Geometry: final body of the model. Coordinates: model frame, mm. A direction names the side the tool comes from. Give positions to 0.01 mm unless a question says otherwise; leave off trailing zeros. Loops run counter-clockwise (first coordinate to the right, second up) from the corner with the lowest first, then second, coordinate; pieces in that order, holes last. Notation, with made-up numbers: (69.5, 26) - (85.5, 26) arc R8 cw to (85.5, 30) - close; hole circle Ø1 at (66.5, -6.5). An arc over 180 degrees is marked (long way). Answer in a Markdown table with one row per item.
from build123d import *

# Parameters (mm, degrees)
CYLINDER004_R     = 2.4
CYLINDER004_DEPTH = 35
CYLINDER011_R     = 2
CYLINDER011_DEPTH = 40
CYLINDER008_R     = 3.15
CYLINDER008_DEPTH = 16
BOX006_W          = 10
BOX006_H          = 24
BOX006_DEPTH      = 15
CHAMFER004_SIZE   = 3
CHAMFER017_SIZE   = 0.4
BOX004_W          = 7
BOX004_H          = 7.8
BOX004_DEPTH      = 8
CHAMFER010_SIZE   = 0.4
BOX003_W          = 18
BOX003_H          = 42
BOX003_DEPTH      = 8
CHAMFER_SIZE      = 7
CHAMFER015_SIZE   = 10
FILLET004_R       = 1
BOX_W             = 1
BOX_H             = 7.8
BOX_DEPTH         = 15


with BuildPart() as cylinder004:
    # Cylinder004 → Cylinder004 (new body)
    with BuildSketch(Plane(origin=(9, 15, 0), x_dir=(1, 0, 0), z_dir=(0, 0, 1))):
        Circle(CYLINDER004_R)
    extrude(amount=CYLINDER004_DEPTH)


with BuildPart() as cylinder011:
    # Cylinder011 → Cylinder011 (new body)
    with BuildSketch(Plane(origin=(9, 34, 2), x_dir=(1, 0, 0), z_dir=(0, 0, 1))):
        Circle(CYLINDER011_R)
    extrude(amount=CYLINDER011_DEPTH)


with BuildPart() as cylinder008:
    # Cylinder008 → Cylinder008 (new body)
    with BuildSketch(Plane(origin=(-2, 15, -7.5), x_dir=(0, 0, -1), z_dir=(1, 0, 0))):
        Circle(CYLINDER008_R)
    extrude(amount=CYLINDER008_DEPTH)


with BuildPart() as chamfer017:
    # Box006 → Box006 (new body)
    with BuildSketch(Plane(origin=(0, 3, -15), x_dir=(1, 0, 0), z_dir=(0, 0, 1))):
        with Locations((5, 12)):
            Rectangle(BOX006_W, BOX006_H)
    extrude(amount=BOX006_DEPTH)

    # Chamfer004
    chamfer004_edges = [chamfer017.edges().sort_by_distance(p)[0] for p in [
        (5, 3, -15),
        (5, 27, -15),
    ]]
    chamfer(chamfer004_edges, length=CHAMFER004_SIZE)

    # Chamfer017
    chamfer017_edges = [chamfer017.edges().sort_by_distance(p)[0] for p in [
        (10, 3, -6),
        (10, 4.5, -13.5),
        (10, 15, -15),
        (10, 27, -6),
        (10, 25.5, -13.5),
    ]]
    chamfer(chamfer017_edges, length=CHAMFER017_SIZE)


with BuildPart() as chamfer010:
    # Box004 → Box004 (new body)
    with BuildSketch(Plane(origin=(-7, 11.1, 0), x_dir=(1, 0, 0), z_dir=(0, 0, 1))):
        with Locations((3.5, 3.9)):
            Rectangle(BOX004_W, BOX004_H)
    extrude(amount=BOX004_DEPTH)

    # Chamfer010
    chamfer010_edges = [chamfer010.edges().sort_by_distance(p)[0] for p in [
        (-7, 11.1, 4),
        (-7, 18.9, 4),
    ]]
    chamfer(chamfer010_edges, length=CHAMFER010_SIZE)


with BuildPart() as fillet004:
    # Box003 → Box003 (new body)
    with BuildSketch(Plane(origin=(0, 3, 0), x_dir=(1, 0, 0), z_dir=(0, 0, 1))):
        with Locations((9, 21)):
            Rectangle(BOX003_W, BOX003_H)
    extrude(amount=BOX003_DEPTH)

    # Chamfer
    chamfer_edges = [fillet004.edges().sort_by_distance(p)[0] for p in [
        (18, 3, 4),
    ]]
    chamfer(chamfer_edges, length=CHAMFER_SIZE)

    # Chamfer015
    chamfer015_edges = [fillet004.edges().sort_by_distance(p)[0] for p in [
        (18, 45, 4),
    ]]
    chamfer(chamfer015_edges, length=CHAMFER015_SIZE)

    # Fillet004
    fillet004_edges = [fillet004.edges().sort_by_distance(p)[0] for p in [
        (18, 35, 4),
        (18, 10, 4),
        (8, 45, 4),
        (11, 3, 4),
    ]]
    fillet(fillet004_edges, radius=FILLET004_R)


with BuildPart() as cut002002002007:
    # Box → Box (new body)
    with BuildSketch(Plane(origin=(-1, 11.1, -15), x_dir=(1, 0, 0), z_dir=(0, 0, 1))):
        with Locations((0.5, 3.9)):
            Rectangle(BOX_W, BOX_H)
    extrude(amount=BOX_DEPTH)

    # Fusion006003: union Chamfer017, Chamfer010, Fillet004
    add(chamfer017.part)
    add(chamfer010.part)
    add(fillet004.part)

    # Cut002002002003: cut Cylinder008
    add(cylinder008.part, mode=Mode.SUBTRACT)

    # Cut002002002006: cut Cylinder011
    add(cylinder011.part, mode=Mode.SUBTRACT)

    # Cut002002002007: cut Cylinder004
    add(cylinder004.part, mode=Mode.SUBTRACT)


solid = cut002002002007.part
Q1. First-contact query: pin 1 (3.5 mm diameter, centred on x = -1.5, z = -6, fed in from +Y); pin 2 (3 mm diameter, centred on x = -3, y = 14, fed in from -Z); pin 3 (1.7 mm diameter, centred on x = 8, y = 15, fed in from +Z). Flat tips, straight axial feed; report the tip coordinate or a pass-through.
Check values:
| item | result |
|---|---|
| pin 1 | y = 27 |
| pin 2 | z = 0 |
| pin 3 | z = 0 |
Q2. Cut plane C-C (y = 14). Output: boundary loops of the cut face in (x, z).
Check values:
| item | result |
|---|---|
| outline | (-7, 0) - (-1, 0) - (-1, -4.51) - (10, -4.51) - (10, 0) - (6.82, 0) - (6.82, 8) - (-7, 8) - close; (-1, -15) - (9.6, -15) - (10, -14.6) - (10, -10.49) - (-1, -10.49) - close; (11.18, 0) - (18, 0) - (18, 8) - (11.18, 8) - close |
Q3. Cut plane B-B (x = 9). Output: boundary loops of the cut face in (y, z).
Check values:
| item | result |
|---|---|
| outline | (3, -12) - (6, -15) - (24, -15) - (27, -12) - (27, 0) - (44, 0) - (44, 8) - (36, 8) - (36, 2) - (32, 2) - (32, 8) - (17.4, 8) - (17.4, 0) - (12.6, 0) - (12.6, 8) - (3, 8) - close; hole circle Ø6.3 at (15, -7.5) |
Q4. Cut plane D-D (y = 34). Output: boundary loops of the cut face in (x, z), and give its area (3 significant figures).
Check values:
| item | result |
|---|---|
| outline | (0, 0) - (18, 0) - (18, 8) - (11, 8) - (11, 2) - (7, 2) - (7, 8) - (0, 8) - close |
| area | 120 mm² |
Q5. Reachability of faces 1 (the cylindrical face through (9, 32, 5)), 2 (the flat face through (0, 29, 1)), 3 (the flat face through (-3, 11.1, 1)), 4 (the flat face through (-4, 15, 0)) from +Z, -Z, +X, -X, +Y, -Y: full face, straight path, thin tool, end or side. Return the list, or none.
Check values:
| item | result |
|---|---|
| face 1 | +Z |
| face 2 | +Z, -Z, -X, +Y |
| face 3 | +Z, -Z, -X, -Y |
| face 4 | -Z, -X, +Y, -Y |
Q6. Draft query along Y for faces 5 (the flat face through (0, 7, -4)), 6 (the flat face through (9, 15, 0)), 7 (the flat face through (-3, 18.9, 1)), 8 (the cylindrical face through (7.23, 16.62, 3.94)). Return one class per face: pulls with the +Y half, pulls with the -Y half, needs draft (parallel to the pull), parting line crosses it, or undercut.
Check values:
| item | result |
|---|---|
| face 5 | needs draft |
| face 6 | undercut |
| face 7 | pulls with the +Y half |
| face 8 | undercut |
Q7. Cut plane A-A (z = -7.5). Output: boundary loops of the cut face in (x, y), and give its area (3 significant figures).
Check values:
| item | result |
|---|---|
| outline | (-1, 11.1) - (0, 11.1) - (0, 3) - (9.6, 3) - (10, 3.4) - (10, 11.85) - (-1, 11.85) - close; (-1, 18.15) - (10, 18.15) - (10, 26.6) - (9.6, 27) - (0, 27) - (0, 18.9) - (-1, 18.9) - close |
| area | 178 mm² |
Q8. Material intervals for line 1 along Z through (x, y) = (4.75, 15); line 2 along Y through (x, z) = (9, 3.6); line 3 along X through (y, z) = (15, 4.75), sorted ascending.
Check values:
| item | result |
|---|---|
| line 1 | -15 to -10.65, -4.35 to 8 |
| line 2 | 3 to 12.6, 17.4 to 32, 36 to 44 |
| line 3 | -7 to 6.6, 11.4 to 18 |
